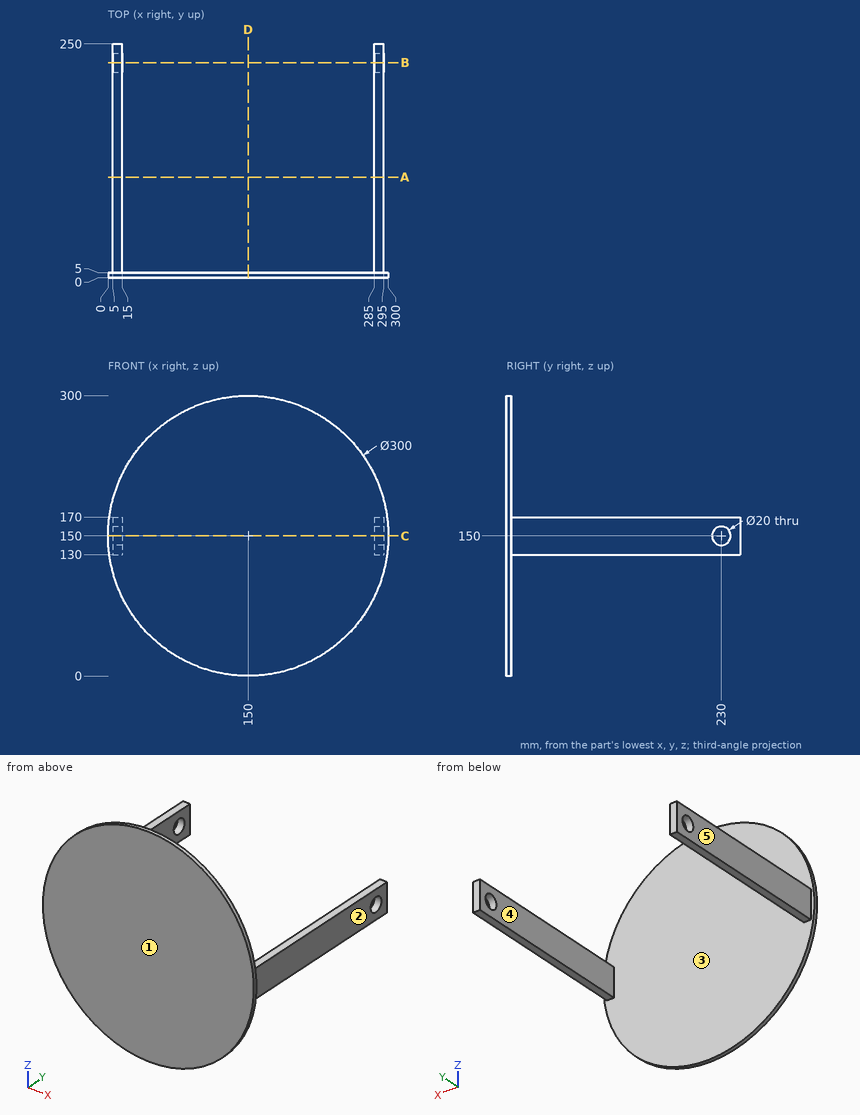
The figure shows three views and two pictorial views of one solid part (mm, origin at its lowest corner). Answer the questions. A direction names the side the tool comes from. Coordinates: 2 decimals unless noted, no trailing zeros. Loops run counter-clockwise (first coordinate to the right, second up) from the corner with the lowest first, then second, coordinate; pieces in that order, holes last. Notation, with made-up numbers: (-39, 84) -> (-3, 84) arc R8 ccw to (-3, 98) -> close; hole circle Ø11 at (-37.75, -36.5). An arc over 180 degrees is marked (long way). Write item = value, one per line. Start each with the question number.
1) The mould has two halves that part along X. Classify the marked faces 1, 2 and 3: released by +X, released by -X, zero draft, split by the parting line, or undercut.
2) Straight lines are drawn through the part: line 1 (X direction, y = 115, z = 152.5); line 2 (Y direction, x = 291, z = 150); line 3 (Y direction, x = 208.5, z = 144.5). For each, find the intervals that lie inside material, in ascending order. Write a range as from..to.
3) A tool of negligible diameter and unlimited length cuts with its end or side. For the marked faces 4 and 5, from which of +Z, -Z, +X, -X, +Y, -Y can it reach the whole face along a straight path? Write none if from no direction.
4) A cutting plane is placed at D-D (x = 150). Give the vertices of the cut face in (y, z).
5) A cutting plane is placed at B-B (y = 230). Give the vertices of the cut face in (x, z), then the cut area to 3 significant figures.
6) A cutting plane is placed at A-A (y = 107.5). Give the vertices of the cut face in (x, z), then the cut area to 3 significant figures.
7) A cutting plane is placed at C-C (z = 150). Give the vertices of the cut face in (x, y).
8) Given pin 1 Ø3 at (x, y) = (291.5, 178.5) entering from -Z; pin 2 Ø11 at (x, y) = (9.5, 112) entering from +Z; pin 3 Ø4 at (x, z) = (180, 43.5) entering from +Y, each flat-ended and moving along its own axis, determine where each tip first touches the part or whether it passes through.
Responses:
q1.face_1 = zero draft
q1.face_2 = released by +X
q1.face_3 = undercut
q2.line_1 = 5..15, 285..295
q2.line_2 = 0..220, 240..250
q2.line_3 = 0..5
q3.face_4 = +Z, -Z, +Y
q3.face_5 = +Z, -Z, -X, +Y
q4.outline = (0, 0) -> (5, 0) -> (5, 300) -> (0, 300) -> close
q5.outline = (5, 130) -> (15, 130) -> (15, 140) -> (5, 140) -> close; (5, 160) -> (15, 160) -> (15, 170) -> (5, 170) -> close; (285, 130) -> (295, 130) -> (295, 140) -> (285, 140) -> close; (285, 160) -> (295, 160) -> (295, 170) -> (285, 170) -> close
q5.area = 400 mm²
q6.outline = (5, 130) -> (15, 130) -> (15, 170) -> (5, 170) -> close; (285, 130) -> (295, 130) -> (295, 170) -> (285, 170) -> close
q6.area = 800 mm²
q7.outline = (0, 0) -> (300, 0) -> (300, 5) -> (295, 5) -> (295, 220) -> (285, 220) -> (285, 5) -> (15, 5) -> (15, 220) -> (5, 220) -> (5, 5) -> (0, 5) -> close; (5, 240) -> (15, 240) -> (15, 250) -> (5, 250) -> close; (285, 240) -> (295, 240) -> (295, 250) -> (285, 250) -> close
q8.pin_1 = 130
q8.pin_2 = 170
q8.pin_3 = 5
